CAD build for the part. Positions are in the model's coordinates, mm. Face numbers are marked on the shaded views. A direction names the side the tool comes from. Coordinates: 2 decimals unless noted, no trailing zeros. Order: outer loops, then holes, each group sorted by start corner. A loop starts at its lowest first (then second) coordinate and runs counter-clockwise, first axis right, second up. Notation, with made-up numbers: M 69.25,-32.75 L 112.25,-32.75 A20 cw 112.25,-12.75 Z; hole C 21,54.25 d7. An arc over 180 degrees is marked long. One line per item, written item: value.
from build123d import *

# Parameters (mm, degrees)
SKETCH1_R           = 1.6
BOSS_EXTRUDE1_DEPTH = 8
CHAMFER1_SIZE       = 1
SKETCH2_R           = 1.6
BOSS_EXTRUDE3_DEPTH = 8
FILLET1_R           = 2
CHAMFER3_SIZE       = 1
CHAMFER4_SIZE       = 1
CHAMFER5_SIZE       = 1


with BuildPart() as part:
    # Sketch1 → Boss-Extrude1 (new body)
    with BuildSketch(Plane.XY):
        with BuildLine():
            Line((-0.5, 3), (60.5, 3))
            ThreePointArc((60.5, 3), (62.267766953, 2.267766953), (63, 0.5))
            Line((63, 0.5), (63, -0.5))
            ThreePointArc((63, -0.5), (62.267766953, -2.267766953), (60.5, -3))
            Line((60.5, -3), (-0.5, -3))
            ThreePointArc((-0.5, -3), (-2.267766953, -2.267766953), (-3, -0.5))
            Line((-3, -0.5), (-3, 0.5))
            ThreePointArc((-3, 0.5), (-2.267766953, 2.267766953), (-0.5, 3))
        make_face()
        Circle(SKETCH1_R, mode=Mode.SUBTRACT)
        with Locations((7.5, 0)):
            Circle(SKETCH1_R, mode=Mode.SUBTRACT)
        with Locations((15, 0)):
            Circle(SKETCH1_R, mode=Mode.SUBTRACT)
        with Locations((22.5, 0)):
            Circle(SKETCH1_R, mode=Mode.SUBTRACT)
        with Locations((30, 0)):
            Circle(SKETCH1_R, mode=Mode.SUBTRACT)
        with Locations((37.5, 0)):
            Circle(SKETCH1_R, mode=Mode.SUBTRACT)
        with Locations((45, 0)):
            Circle(SKETCH1_R, mode=Mode.SUBTRACT)
        with Locations((52.5, 0)):
            Circle(SKETCH1_R, mode=Mode.SUBTRACT)
        with Locations((60, 0)):
            Circle(SKETCH1_R, mode=Mode.SUBTRACT)
    extrude(amount=BOSS_EXTRUDE1_DEPTH)

    # Chamfer1
    chamfer1_edges = [part.edges().sort_by_distance(p)[0] for p in [
        (-1.6, 0, 0),
        (-1.6, 0, 8),
        (5.9, 0, 0),
        (5.9, 0, 8),
        (13.4, 0, 0),
        (13.4, 0, 8),
        (20.9, 0, 0),
        (20.9, 0, 8),
        (28.4, 0, 0),
        (28.4, 0, 8),
    ]]
    chamfer(chamfer1_edges, length=CHAMFER1_SIZE)

    # Sketch2 → Boss-Extrude3 (add)
    with BuildSketch(Plane.XY.offset(8)):
        with BuildLine():
            ThreePointArc((-0.5, -3), (-2.267766953, -2.267766953), (-3, -0.5))
            Line((-3, -0.5), (-3, -23))
            ThreePointArc((-3, -23), (-2.267766953, -24.767766953), (-0.5, -25.5))
            Line((-0.5, -25.5), (0.5, -25.5))
            ThreePointArc((0.5, -25.5), (2.267766953, -24.767766953), (3, -23))
            Line((3, -23), (3, -3))
            Line((3, -3), (-0.5, -3))
        make_face()
        with Locations((0, -22.5)):
            Circle(SKETCH2_R, mode=Mode.SUBTRACT)
        with Locations((0, -15)):
            Circle(SKETCH2_R, mode=Mode.SUBTRACT)
        with Locations((0, -7.5)):
            Circle(SKETCH2_R, mode=Mode.SUBTRACT)
    extrude(amount=-BOSS_EXTRUDE3_DEPTH)

    # Fillet1
    fillet1_edges = [part.edges().sort_by_distance(p)[0] for p in [
        (3, -3, 4),
    ]]
    fillet(fillet1_edges, radius=FILLET1_R)

    # Chamfer3
    chamfer3_edges = [part.edges().sort_by_distance(p)[0] for p in [
        (35.9, 0, 0),
        (35.9, 0, 8),
        (43.4, 0, 0),
        (43.4, 0, 8),
    ]]
    chamfer(chamfer3_edges, length=CHAMFER3_SIZE)

    # Chamfer4
    chamfer4_edges = [part.edges().sort_by_distance(p)[0] for p in [
        (50.9, 0, 0),
        (50.9, 0, 8),
        (58.4, 0, 0),
        (58.4, 0, 8),
    ]]
    chamfer(chamfer4_edges, length=CHAMFER4_SIZE)

    # Chamfer5
    chamfer5_edges = [part.edges().sort_by_distance(p)[0] for p in [
        (-1.6, -7.5, 8),
        (-1.6, -15, 8),
        (-1.6, -22.5, 8),
        (-1.6, -22.5, 0),
        (-1.6, -15, 0),
        (-1.6, -7.5, 0),
    ]]
    chamfer(chamfer5_edges, length=CHAMFER5_SIZE)


solid = part.part
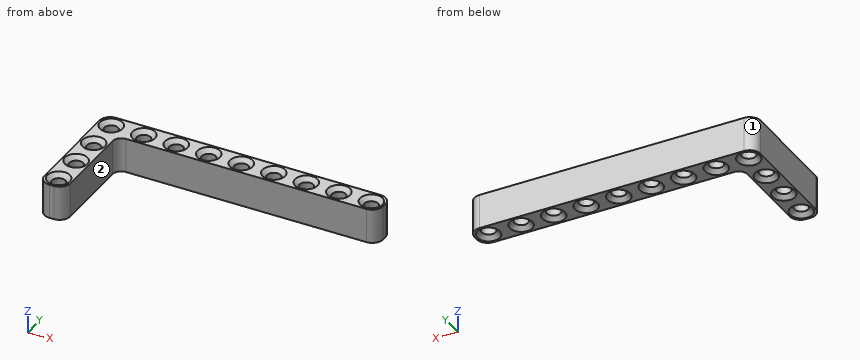
Q1. Drill centre lines: line 1 along Y through (x, z) = (0, 3.95); line 2 along Y through (x, z) = (1, 6.25); line 3 along Y through (x, z) = (15, 3.55). Where is each one in solid material? Low to high.
Recorded:
line 1: y = -25.5 to -24.1, -20.9 to -16.6, -13.4 to -9.1, -5.9 to -1.6, 1.6 to 3
line 2: y = -25.45 to -23.75, -21.25 to -16.25, -13.75 to -8.75, -6.25 to -1.25, 1.25 to 3
line 3: y = -3 to -1.6, 1.6 to 3
Q2. Pin check, flat tips, straight feed: pin 1 Ø4 at (x, z) = (52, 5.5) entering from -Y; pin 2 Ø3 at (y, z) = (-3, 3.5) entering from +X; pin 3 Ø1.9 at (x, y) = (52.5, 0) entering from +Z; pin 4 Ø3.5 at (x, y) = (45, 0) entering from +Z. Stop position of each tip, or through.
Recorded:
pin 1: stops at y = -3
pin 2: stops at x = 62.79
pin 3: passes through
pin 4: stops at z = 7.15
Q3. Which spindle directions (+Z, -Z, +X, -X, +Y, -Y) get a long thin tool onto all of the face, cutting with end or side? Do the marked faces 1 and 2. Say none if no direction does.
Recorded:
face 1: +Z, -Z, -X, +Y
face 2: +Z, -Z, +X, -Y
Q4. Slice it at B-B (z = 4.5). Give the number of separate pieces and of enclosed holes in the cut face, plus the area to 3 significant figures.
Recorded:
separate pieces: 1
enclosed holes: 12
area: 429 mm^2
Q5. Slice it at A-A (x = 52.5). List the corners of the cut face in (y, z), plus the area to 3 significant figures.
Recorded:
outline: M -3,0 L -2.6,0 L -1.6,1 L -1.6,7 L -2.6,8 L -3,8 Z; M 1.6,1 L 2.6,0 L 3,0 L 3,8 L 2.6,8 L 1.6,7 Z
area: 20.4 mm^2
